Verification items for the finished model (mm, model axes). Face numbers are marked on the shaded views. A direction names the side the tool comes from. Coordinates: 2 decimals unless noted, no trailing zeros. Order: outer loops, then holes, each group sorted by start corner. A loop starts at its lowest first (then second) coordinate and runs counter-clockwise, first axis right, second up. Notation, with made-up numbers: (39, 71.5) - (82, 71.5) arc R26 ccw to (82, 99.5) - close; hole circle Ø10 at (84.25, 41). An arc over 180 degrees is marked (long way). Answer as CSV lines item,"result". Start each with the question number.
1. Material ranges on L1, parallel to X at y = 7.5, z = -19.75; L2, parallel to Z at x = 21.5, y = -23.5; L3, parallel to Z at x = 7, y = -27, recorded low to high. Write a range as [from, to].
2. Mould release check, pull along Z, two halves, no side actions. Record for the marked faces 4, 5 and 6: pulls with the +Z half, pulls with the -Z half, needs draft (parallel to the pull), parting line crosses it, or undercut.
3. Section check A-A (z = -24.75). Record the cut outline in (x, y), and give its area (3 significant figures).
4. Go/stop test with flat-tipped pins: pin 1 (16 mm diameter, centred on y = -22, z = -16, fed in from -X); pin 2 (7 mm diameter, centred on y = -1.15, z = -18, fed in from +X); pin 3 (6 mm diameter, centred on y = 0, z = -18.5, fed in from +X); pin 4 (1.5 mm diameter, centred on y = -0.5, z = -3.5, fed in from -X). Record where each tip stops, or that it passes through.
5. Section check C-C (x = 30). Record the cut outline in (y, z).
6. Section check B-B (y = -9). Record the cut outline in (x, z), and give its area (3 significant figures).
7. Set-up check for the marked faces 1, 2 and 3: record each of +Z, -Z, +X, -X, +Y, -Y from which the full face is reachable in a straight line by a thin tool's end or side.
8. Section check D-D (y = 1). Count the separate pieces of the cut face and the enclosed holes in it, and give its area (3 significant figures).
from build123d import *

# Parameters (mm, degrees)
F0_W     = 48
F0_H     = 28
F1_DEPTH = 36
F2_W     = 20
F2_H     = 48
F3_DEPTH = 20
F4_R     = 5
F5_R     = 4
F6_DEPTH = 36
F7_R     = 6
F8_DEPTH = 4
F9_SIZE  = 1


with BuildPart() as f1:
    # F0 (on Right) → F1 (new body)
    with BuildSketch(Plane.YZ):
        with Locations((-13.1489487588, -14)):
            Rectangle(F0_W, F0_H)
    extrude(amount=F1_DEPTH)

    # F2 (on face) → F3 (cut)
    with BuildSketch(Plane(origin=(0, 0, -28), x_dir=(1, 0, 0), z_dir=(0, 0, -1))):
        with Locations((18, 13.1489487588)):
            Rectangle(F2_W, F2_H)
    extrude(amount=-F3_DEPTH, mode=Mode.SUBTRACT)

    # F4
    f4_edges = [f1.edges().sort_by_distance(p)[0] for p in [
        (0, -13.148949, 0),
        (36, -13.148949, 0),
    ]]
    fillet(f4_edges, radius=F4_R)

    # F5 (on face) → F6 (cut)
    with BuildSketch(Plane.YZ.offset(36)):
        with Locations((46.8510512412, -18)):
            Circle(F5_R)
        with Locations((22.8510512412, -18)):
            Circle(F5_R)
        with Locations((-1.1489487588, -18)):
            Circle(F5_R)
        with Locations((-25.1489487588, -18)):
            Circle(F5_R)
    extrude(amount=-F6_DEPTH, mode=Mode.SUBTRACT)

    # F7 (on face) → F8 (cut)
    with BuildSketch(Plane.YZ.offset(36)):
        with Locations((-25.1489487588, -18)):
            Circle(F7_R)
        with Locations((-1.1489487588, -18)):
            Circle(F7_R)
        with Locations((22.8510512412, -18)):
            Circle(F7_R)
        with Locations((46.8510512412, -18)):
            Circle(F7_R)
    extrude(amount=-F8_DEPTH, mode=Mode.SUBTRACT)

    # F9
    f9_edges = [f1.edges().sort_by_distance(p)[0] for p in [
        (32, -29.148949, -18),
        (32, -5.148949, -18),
    ]]
    chamfer(f9_edges, length=F9_SIZE)


solid = f1.part
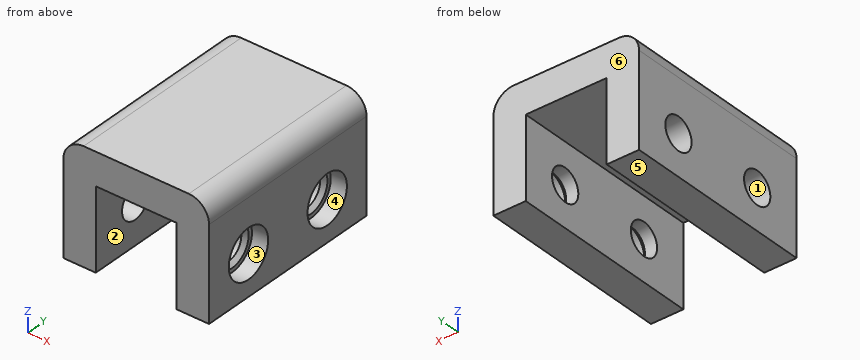
Evaluation:
1,L1,"x = [0, 8], [28, 36]"
1,L2,"z = [-8, 0]"
1,L3,"z = [-28, -21.55], [-14.45, 0]"
2,face 4,"undercut"
2,face 5,"pulls with the -Z half"
2,face 6,"needs draft"
3,outline,"(0, -37.15) - (8, -37.15) - (8, 10.85) - (0, 10.85) - close; (28, -37.15) - (36, -37.15) - (36, 10.85) - (28, 10.85) - close"
3,area,"768 mm²"
4,pin 1,"stops at x = 0"
4,pin 2,"passes through"
4,pin 3,"stops at x = 31.25"
4,pin 4,"stops at x = 0.06"
5,outline,"(-37.15, -28) - (10.85, -28) - (10.85, 0) - (-37.15, 0) - close; hole circle Ø8 at (-25.15, -18); hole circle Ø8 at (-1.15, -18)"
6,outline,"(0, -28) - (8, -28) - (8, -8) - (28, -8) - (28, -28) - (36, -28) - (36, -5) arc R5 ccw to (31, 0) - (5, 0) arc R5 ccw to (0, -5) - close"
6,area,"597 mm²"
7,face 1,"+X, -X"
7,face 2,"-Z, +Y, -Y"
7,face 3,"+X"
8,separate pieces,"3"
8,enclosed holes,"0"
8,area,"470 mm²"
